```python
from build123d import *

# Parameters (mm, degrees)
SKETCH1_R           = 30
BOSS_EXTRUDE1_DEPTH = 6.35
FILLET1_R           = 3.175
SKETCH2_W           = 6.3754
SKETCH2_H           = 6.3754
CUT_EXTRUDE1_DEPTH  = 17.462


with BuildPart() as part:
    # Sketch1 → Boss-Extrude1 (new body)
    with BuildSketch(Plane.XY):
        Circle(SKETCH1_R)
        with BuildLine():
            Line((-2, 24.919871589), (-2, 6.026815079))
            ThreePointArc((-2, 6.026815079), (-3.175, 5.499261314), (-4.219374963, 4.745458347))
            Line((-4.219374963, 4.745458347), (-20.581241855, 14.191986602))
            ThreePointArc((-20.581241855, 14.191986602), (-12.5, 21.650635095), (-2, 24.919871589))
        make_face(mode=Mode.SUBTRACT)
        with BuildLine():
            Line((-22.581241855, 10.727884987), (-6.219374963, 1.281356732))
            ThreePointArc((-6.219374963, 1.281356732), (-6.35, 0), (-6.219374963, -1.281356732))
            Line((-6.219374963, -1.281356732), (-22.581241855, -10.727884987))
            ThreePointArc((-22.581241855, -10.727884987), (-25, 0), (-22.581241855, 10.727884987))
        make_face(mode=Mode.SUBTRACT)
        with BuildLine():
            Line((-20.581241855, -14.191986602), (-4.219374963, -4.745458347))
            ThreePointArc((-4.219374963, -4.745458347), (-3.175, -5.499261314), (-2, -6.026815079))
            Line((-2, -6.026815079), (-2, -24.919871589))
            ThreePointArc((-2, -24.919871589), (-12.5, -21.650635095), (-20.581241855, -14.191986602))
        make_face(mode=Mode.SUBTRACT)
        with BuildLine():
            Line((2, -24.919871589), (2, -6.026815079))
            ThreePointArc((2, -6.026815079), (3.175, -5.499261314), (4.219374963, -4.745458347))
            Line((4.219374963, -4.745458347), (20.581241855, -14.191986602))
            ThreePointArc((20.581241855, -14.191986602), (12.5, -21.650635095), (2, -24.919871589))
        make_face(mode=Mode.SUBTRACT)
        with BuildLine():
            Line((22.581241855, -10.727884987), (6.219374963, -1.281356732))
            ThreePointArc((6.219374963, -1.281356732), (6.35, 0), (6.219374963, 1.281356732))
            Line((6.219374963, 1.281356732), (22.581241855, 10.727884987))
            ThreePointArc((22.581241855, 10.727884987), (25, 0), (22.581241855, -10.727884987))
        make_face(mode=Mode.SUBTRACT)
        with BuildLine():
            Line((20.581241855, 14.191986602), (4.219374963, 4.745458347))
            ThreePointArc((4.219374963, 4.745458347), (3.175, 5.499261314), (2, 6.026815079))
            Line((2, 6.026815079), (2, 24.919871589))
            ThreePointArc((2, 24.919871589), (12.5, 21.650635095), (20.581241855, 14.191986602))
        make_face(mode=Mode.SUBTRACT)
    extrude(amount=BOSS_EXTRUDE1_DEPTH)

    # Fillet1
    # the kernel refuses this fillet: 3.175 mm, written as the material it adds along each edge
    with BuildSketch(Plane(origin=(-22.581241855, -10.727884987, 0), x_dir=(-0.3558834781816715, 0.9345303365634076, 0), z_dir=(0, 0, 1)), Plane(origin=(22.581241855, 10.727884987, 0), x_dir=(0.3558834781815518, -0.9345303365634531, 0), z_dir=(0, 0, 1)), Plane(origin=(-20.581241855, 14.191986602, 0), x_dir=(0.63138527298033, 0.7754693011741691, 0), z_dir=(0, 0, 1))) as fillet1_piece_1:
        with BuildLine():
            CenterArc((3.725852278, -3.164933037), FILLET1_R, 85.436166165, 103.716233406)
            Line((0.591273993, -3.669951824), (0, 0))
            ThreePointArc((0, 0), (1.989243074, 0.079267427), (3.978486149, 0))
        make_face()
    extrude(amount=6.35)
    with BuildSketch(Plane(origin=(-22.581241855, 10.727884987, 0), x_dir=(-0.3558834781816212, -0.9345303365634268, 0), z_dir=(0, 0, 1)), Plane(origin=(2, -24.919871589, 0), x_dir=(0.987268751161949, 0.1590610353893298, 0), z_dir=(0, 0, 1)), Plane(origin=(22.581241855, -10.727884987, 0), x_dir=(0.35588347818151106, 0.9345303365634686, 0), z_dir=(0, 0, 1)), Plane(origin=(-2, 24.919871589, 0), x_dir=(-0.9872687511619511, -0.15906103538931676, 0), z_dir=(0, 0, 1))) as fillet1_piece_2:
        with BuildLine():
            CenterArc((3.725852278, 3.164933037), FILLET1_R, 170.847600429, 103.716233406)
            Line((0.591273993, 3.669951824), (0, 0))
            ThreePointArc((0, 0), (1.989243074, -0.079267427), (3.978486149, 0))
        make_face()
    extrude(amount=6.35)
    with BuildSketch(Plane(origin=(-20.581241855, -14.191986602, 0), x_dir=(0.8660254037844406, 0.49999999999999667, 0), z_dir=(0, 0, 1)), Plane(origin=(20.581241855, 14.191986602, 0), x_dir=(-0.8660254037844309, -0.5000000000000133, 0), z_dir=(0, 0, 1))) as fillet1_piece_3:
        with BuildLine():
            CenterArc((3.717277408, -3.175), FILLET1_R, 90, 103.716233406)
            ThreePointArc((0.632822126, -3.927835052), (0.23815281, -1.976525885), (0, 0))
            Line((0, 0), (3.717277408, 0))
        make_face()
    extrude(amount=6.35)
    with BuildSketch(Plane(origin=(-2, -24.919871589, 0), x_dir=(0, 1, 0), z_dir=(0, 0, 1)), Plane(origin=(20.581241855, -14.191986602, 0), x_dir=(-0.8660254037844468, 0.49999999999998584, 0), z_dir=(0, 0, 1)), Plane(origin=(2, 24.919871589, 0), x_dir=(0, -1, 0), z_dir=(0, 0, 1))) as fillet1_piece_4:
        with BuildLine():
            CenterArc((3.717277408, 3.175), FILLET1_R, 166.283766594, 103.716233406)
            ThreePointArc((0.632822126, 3.927835052), (0.23815281, 1.976525885), (0, 0))
            Line((0, 0), (3.717277408, 0))
        make_face()
    extrude(amount=6.35)
    with BuildSketch(Plane(origin=(4.219374963, 4.745458347, 0), x_dir=(0.8660254037844292, 0.5000000000000164, 0), z_dir=(0, 0, 1)), Plane(origin=(6.219374963, -1.281356732, 0), x_dir=(0.8660254037845205, -0.4999999999998582, 0), z_dir=(0, 0, 1)), Plane(origin=(2, -6.026815079, 0), x_dir=(0, -1, 0), z_dir=(0, 0, 1)), Plane(origin=(-2, 6.026815079, 0), x_dir=(0, 1, 0), z_dir=(0, 0, 1)), Plane(origin=(-6.219374963, 1.281356732, 0), x_dir=(-0.866025403784444, 0.49999999999999056, 0), z_dir=(0, 0, 1)), Plane(origin=(-4.219374963, -4.745458347, 0), x_dir=(-0.8660254037844402, -0.49999999999999745, 0), z_dir=(0, 0, 1))) as fillet1_piece_5:
        with BuildLine():
            CenterArc((1.969746682, 3.175), FILLET1_R, 212.909051607, 57.090948393)
            ThreePointArc((-0.695773905, 1.45), (-0.301795458, 0.747116731), (0, 0))
            Line((0, 0), (1.969746682, 0))
        make_face()
    extrude(amount=6.35)
    with BuildSketch(Plane(origin=(2, 6.026815079, 0), x_dir=(0.9015778931723624, -0.43261680797546975, 0), z_dir=(0, 0, 1)), Plane(origin=(6.219374963, 1.281356732, 0), x_dir=(0.07613180077529093, -0.9970977629654534, 0), z_dir=(0, 0, 1)), Plane(origin=(-4.219374963, 4.745458347, 0), x_dir=(0.8254460923970771, 0.5644809549899766, 0), z_dir=(0, 0, 1)), Plane(origin=(-6.219374963, -1.281356732, 0), x_dir=(-0.07613180077550848, 0.9970977629654367, 0), z_dir=(0, 0, 1)), Plane(origin=(-2, -6.026815079, 0), x_dir=(-0.9015778931724164, 0.432616807975357, 0), z_dir=(0, 0, 1))) as fillet1_piece_6:
        with BuildLine():
            CenterArc((2.010364289, 3.149438429), FILLET1_R, 205.633744341, 57.090948393)
            Line((-0.852145522, 1.775880064), (0, 0))
            ThreePointArc((0, 0), (0.804145716, 0.051123142), (1.608291431, 0))
        make_face()
    extrude(amount=6.35)
    with BuildSketch(Plane(origin=(4.219374963, -4.745458347, 0), x_dir=(0.8660254037844309, -0.5000000000000133, 0), z_dir=(0, 0, 1))) as fillet1_piece_7:
        with BuildLine():
            CenterArc((1.969746682, -3.175), FILLET1_R, 90, 57.090948393)
            ThreePointArc((-0.695773905, -1.45), (-0.301795458, -0.747116731), (0, 0))
            Line((0, 0), (1.969746682, 0))
        make_face()
    extrude(amount=6.35)

    # Sketch2 → Cut-Extrude1 (cut)
    with BuildSketch(Plane(origin=(0, 0, 0), x_dir=(-1, 0, 0), z_dir=(0, 0, -1))):
        Rectangle(SKETCH2_W, SKETCH2_H)
    extrude(amount=-CUT_EXTRUDE1_DEPTH, mode=Mode.SUBTRACT)


solid = part.part
```
The listing builds one solid part. Answer for the finished solid, in the listing's coordinates (mm). Coordinates: 2 decimals unless noted, no trailing zeros. Write each loop counter-clockwise with the first axis right and the second up, starting at its lowest first coordinate (ties: lowest second). Pieces come first, ordered by that corner, then holes. Notation, with made-up numbers: (49, -34.75) - (82, -34.75) arc R13 ccw to (82, -17.75) - close; hole circle Ø3 at (-36.75, 77.5). An arc over 180 degrees is marked (long way). Return JSON: item names as keys, results as strings. Group by question number.
1. Determine the mould class of faces 1 (the cylindrical face through (-29.97, 1.32, 3.13)), 2 (the cylindrical face through (6.904, 1.326, 3.131)) for opening direction X: released by +X, released by -X, zero draft, split by the parting line, or undercut.
2. A cutting plane is placed at D-D, the plane x = 13. Determine the outline of the cut face in (y, z).
3. A cutting plane is placed at C-C, the plane z = 1. Give the number of separate pieces and of enclosed holes in the cut face, plus the area to 3 significant figures.
4. A cutting plane is placed at B-B, the plane y = -15.5. Determine the outline of the cut face in (x, z).
5. A cutting plane is placed at A-A, the plane x = 0. Determine the outline of the cut face in (y, z).
6. Straight lines are drawn through the part: L1, parallel to X at y = 9, z = 4.5; L2, parallel to Y at x = -7.5, z = 6.25; L3, parallel to X at y = 2, z = 2. For each, find the intervals that lie inside material, in ascending order.
7. Given pin 1 (2 mm diameter, centred on y = -8.5, z = 2.5, fed in from +X); pin 2 (1.9 mm diameter, centred on y = -17, z = 1.5, fed in from -X), each flat-ended and moving along its own axis, determine where each tip first touches the part or whether it passes through.
Ans:
{
 "1": {"face 1": "split by the parting line", "face 2": "undercut"},
 "2": {"outline": "(-27.04, 0) - (-21.35, 0) - (-21.35, 6.35) - (-27.04, 6.35) - close; (-9.81, 0) - (-5.2, 0) - (-5.2, 6.35) - (-9.81, 6.35) - close; (5.2, 0) - (9.81, 0) - (9.81, 6.35) - (5.2, 6.35) - close; (21.35, 0) - (27.04, 0) - (27.04, 6.35) - (21.35, 6.35) - close"},
 "3": {"separate pieces": "1", "enclosed holes": "7", "area": "1,450 mm²"},
 "4": {"outline": "(-25.69, 0) - (-18.92, 0) - (-18.92, 6.35) - (-25.69, 6.35) - close; (-2, 0) - (2, 0) - (2, 6.35) - (-2, 6.35) - close; (18.92, 0) - (25.69, 0) - (25.69, 6.35) - (18.92, 6.35) - close"},
 "5": {"outline": "(-30, 0) - (-3.19, 0) - (-3.19, 6.35) - (-30, 6.35) - close; (3.19, 0) - (30, 0) - (30, 6.35) - (3.19, 6.35) - close"},
 "6": {"L1": "-28.62 to -22.29, -19.61 to -11.59, -2 to 2, 11.59 to 19.61, 22.29 to 28.62", "L2": "-29.05 to -23.85, -6.64 to -1.97, 1.97 to 6.64, 23.85 to 29.05", "L3": "-29.93 to -24.92, -7.53 to -3.19, 3.19 to 7.53, 24.92 to 29.93"},
 "7": {"pin 1": "x = 29.05", "pin 2": "x = -25.35"}
}
